from build123d import *

# Parameters (mm, degrees)
EXTRUDE_334_DEPTH = 15
SKETCH_2_R        = 30
EXTRUDE_1_DEPTH   = 60
EXTRUDE_2_DEPTH   = 15
SKETCH_4_R        = 10
EXTRUDE_3_DEPTH   = 35
SKETCH_5_R        = 15
EXTRUDE_4_DEPTH   = 25
SKETCH_6_R        = 4
EXTRUDE_5_DEPTH   = 5
EXTRUDE_6_DEPTH   = 100
SKETCH_8_W        = 14
SKETCH_8_H        = 11
EXTRUDE_7_DEPTH   = 20


with BuildPart() as part:
    # Sketch 1 → Extrude 334 (new body)
    with BuildSketch(Plane(origin=(0, 0, 0), x_dir=(0, 0, -1), z_dir=(1, 0, 0))):
        Polygon((0, 28.867513459), (-25, 14.43375673), (-25, -14.43375673), (0, -28.867513459), (25, -14.43375673), (25, 14.43375673), align=None)
    extrude(amount=EXTRUDE_334_DEPTH)

    # Sketch 2 → Extrude 1 (add)
    with BuildSketch(Plane.ZY):
        Circle(SKETCH_2_R)
    extrude(amount=EXTRUDE_1_DEPTH)

    # Sketch 3 → Extrude 2 (add)
    with BuildSketch(Plane.ZY.offset(60)):
        Polygon((0, 28.867513459), (-25, 14.43375673), (-25, -14.43375673), (0, -28.867513459), (25, -14.43375673), (25, 14.43375673), align=None)
    extrude(amount=EXTRUDE_2_DEPTH)

    # Sketch 4 → Extrude 3 (add)
    with BuildSketch(Plane(origin=(0, 0, 0), x_dir=(1, 0, 0), z_dir=(0, 1, 0))):
        with Locations(Location((-30, 0, 0), (0, 0, 90))):
            Circle(SKETCH_4_R)
    extrude(amount=EXTRUDE_3_DEPTH)

    # Sketch 5 → Extrude 4 (add)
    with BuildSketch(Plane(origin=(0, 35, 0), x_dir=(-1, 0, 0), z_dir=(0, 1, 0))):
        with Locations(Location((30, 0, 0), (0, 0, 90))):
            Circle(SKETCH_5_R)
    extrude(amount=EXTRUDE_4_DEPTH)

    # Sketch 6 → Extrude 5 (add)
    with BuildSketch(Plane(origin=(0, 60, 0), x_dir=(-1, 0, 0), z_dir=(0, 1, 0))):
        with Locations(Location((30, 0, 0), (0, 0, 90))):
            Circle(SKETCH_6_R)
    extrude(amount=EXTRUDE_5_DEPTH)

    # Sketch 7 → Extrude 6 (add)
    with BuildSketch(Plane(origin=(-30, 0, 0), x_dir=(0, 0, -1), z_dir=(1, 0, 0))):
        Polygon((-4, 57), (0, 57), (4, 57), (4, 52), (-4, 52), align=None)
    extrude(amount=EXTRUDE_6_DEPTH)

    # Sketch 8 → Extrude 7 (add)
    with BuildSketch(Plane(origin=(70, 0, 0), x_dir=(0, 0, -1), z_dir=(1, 0, 0))):
        with Locations((0, 54.5)):
            Rectangle(SKETCH_8_W, SKETCH_8_H)
    extrude(amount=-EXTRUDE_7_DEPTH)


solid = part.part
Build history of the part. All positions in model axes, mm. A direction names the side the tool comes from. Coordinates: 2 decimals unless noted, no trailing zeros. Order: outer loops, then holes, each group sorted by start corner. A loop starts at its lowest first (then second) coordinate and runs counter-clockwise, first axis right, second up. Notation, with made-up numbers: (-29.5, 57) -> (18.5, 57) arc R11 ccw to (18.5, 69) -> close; hole circle Ø5 at (71.5, 36). An arc over 180 degrees is marked (long way). One line per item, written item: value.
(1) Slice it at D-D, the plane x = 42.5. List the corners of the cut face in (y, z), plus the area to 3 significant figures.
Checked values:
outline: (52, -4) -> (57, -4) -> (57, 4) -> (52, 4) -> close
area: 40.0 mm2
(2) Tool access for faces 1 (the flat face through (-33, 60, 3)), 2 (the flat face through (7, 0, 25)), 3 (the flat face through (-60, 20.14, 15.42)): list every direction of +Z, -Z, +X, -X, +Y, -Y with a clear straight run to the whole face (end or side of a thin tool).
Checked values:
face 1: +Y
face 2: +Z, +X, +Y, -Y
face 3: -X
(3) Mould opens along X. For faces 4 (the cylindrical face through (-33, 32.34, -9.54)), 5 (the flat face through (17, 57, 0)), 6 (the flat face through (7.4, 21.75, 12.33)), 7 (the flat face through (50, 58, 0)) say: pulls with the +X half, pulls with the -X half, needs draft (parallel to the pull), parting line crosses it, or undercut.
Checked values:
face 4: parting line crosses it
face 5: undercut
face 6: needs draft
face 7: undercut
(4) Slice it at A-A, the plane x = -30. List the corners of the cut face in (y, z).
Checked values:
outline: (28.28, -10) -> (35, -10) -> (35, -15) -> (60, -15) -> (60, -4) -> (65, -4) -> (65, 4) -> (60, 4) -> (60, 15) -> (35, 15) -> (35, 10) -> (28.28, 10) arc R30 ccw (long way) to start
(5) Probe line 1 (X direction, y = 6, z = -24); line 2 (Y direction, x = -43, z = 0.5); line 3 (Y direction, x = 32, z = -0.5). List the from-to ranges inside material, lowest first. Write a range as [from, to].
Checked values:
line 1: [-75, 15]
line 2: [-30, 30], [35, 60]
line 3: [52, 57]
(6) Slice it at C-C, the plane z = -5.5. List the corners of the cut face in (x, y).
Checked values:
outline: (-75, -25.69) -> (-60, -25.69) -> (-60, -29.49) -> (0, -29.49) -> (0, -25.69) -> (15, -25.69) -> (15, 25.69) -> (0, 25.69) -> (0, 29.49) -> (-21.65, 29.49) -> (-21.65, 35) -> (-16.04, 35) -> (-16.04, 60) -> (-43.96, 60) -> (-43.96, 35) -> (-38.35, 35) -> (-38.35, 29.49) -> (-60, 29.49) -> (-60, 25.69) -> (-75, 25.69) -> close; (50, 49) -> (70, 49) -> (70, 60) -> (50, 60) -> close
(7) Drop flat-ended pins along their axis: pin 1 Ø6 at (y, z) = (52, 11) entering from +X; pin 2 Ø7 at (x, z) = (60.5, -3) entering from +Y; pin 3 Ø4 at (x, z) = (62, 1) entering from -Y. Give the stop position or say it passes through.
Checked values:
pin 1: x = -17.31
pin 2: y = 60
pin 3: y = 49
(8) Slice it at B-B, the plane y = 0. List the corners of the cut face in (x, z).
Checked values:
outline: (-75, -25) -> (-60, -25) -> (-60, -30) -> (0, -30) -> (0, -25) -> (15, -25) -> (15, 25) -> (0, 25) -> (0, 30) -> (-60, 30) -> (-60, 25) -> (-75, 25) -> close
